Print and shaded views of the part. All mm, measured from the part's lowest x, y and z. Round coordinates to 2 decimals unless told otherwise and drop trailing zeros. Loops run counter-clockwise (first coordinate to the right, second up) from the corner with the lowest first, then second, coordinate; pieces in that order, holes last. Notation, with made-up numbers: (-20.5, 62) - (25.5, 62) arc R22 ccw to (25.5, 95) - close; hole circle Ø4 at (26, -37). An arc over 180 degrees is marked (long way). Use one line per item in the form item = value.
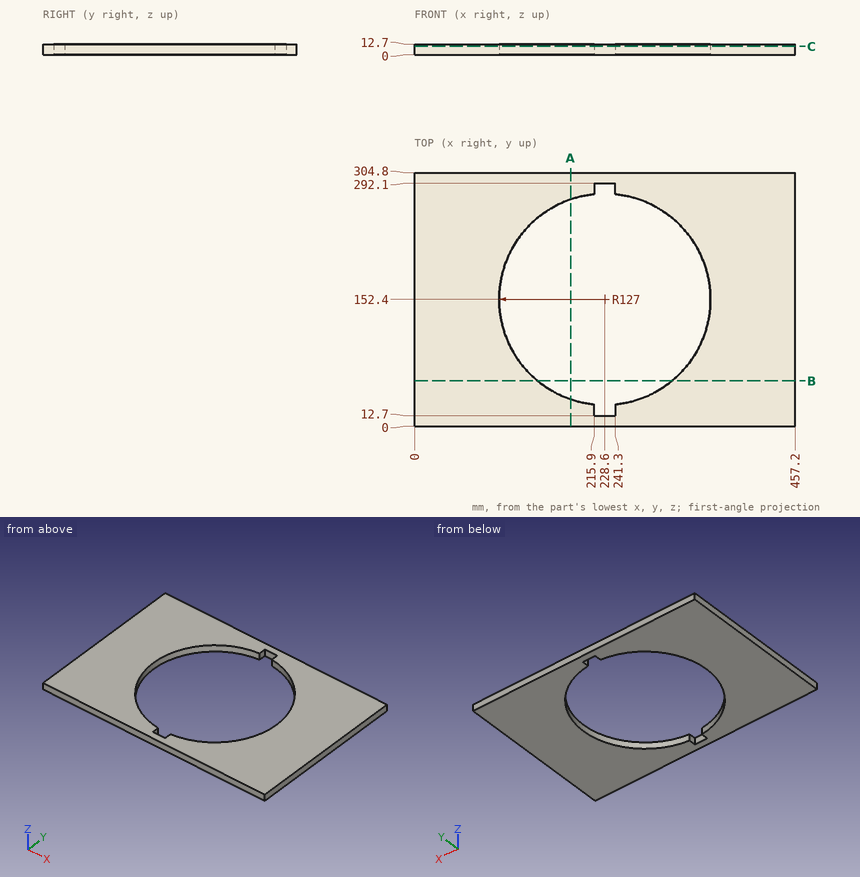
1) Slice it at C-C (z = 9.75). Write the cut outline in (x, y).
Report:
outline = (0, 0) - (457.2, 0) - (457.2, 304.8) - (0, 304.8) - close; hole (215.9, 12.7) - (241.3, 12.7) - (241.3, 26.04) arc R127 ccw to (241.3, 278.76) - (241.3, 292.1) - (215.9, 292.1) - (215.9, 278.76) arc R127 ccw to (215.9, 26.04) - close
2) Drill centre lines: probe 1 along X at (y, z) = (14, 6.5); probe 2 along Y at (x, z) = (240, 9.25); probe 3 along X at (y, z) = (115, 10.5). Where is each one in solid material? Low to high.
Report:
probe_1 = 0 to 215.9, 241.3 to 457.2
probe_2 = 0 to 12.7, 292.1 to 304.8
probe_3 = 0 to 107.23, 349.97 to 457.2
3) Slice it at B-B (y = 54.5). Write the cut outline in (x, z).
Report:
outline = (0, 0) - (147.7, 0) - (147.7, 12.7) - (0, 12.7) - close; (309.5, 0) - (457.2, 0) - (457.2, 12.7) - (309.5, 12.7) - close
4) Slice it at A-A (x = 187.5). Write the cut outline in (y, z), plus the area to 3 significant figures.
Report:
outline = (0, 0) - (32.23, 0) - (32.23, 12.7) - (0, 12.7) - close; (272.57, 0) - (304.8, 0) - (304.8, 12.7) - (272.57, 12.7) - close
area = 819 mm^2
